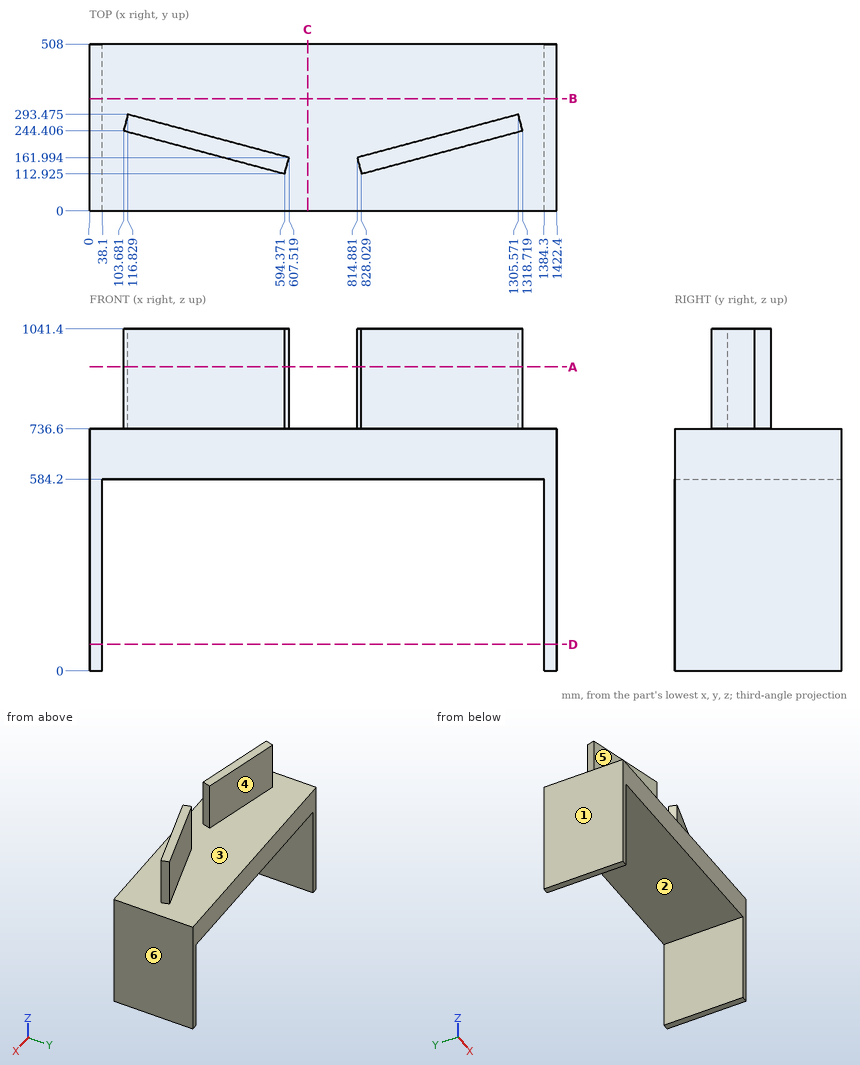
For this review, use the dimensioned drawing (mm, ordinates from the lowest corner) and the shaded views. A direction names the side the tool comes from. Round coordinates to 2 decimals unless told otherwise and drop trailing zeros. Order: outer loops, then holes, each group sorted by start corner. A loop starts at its lowest first (then second) coordinate and runs counter-clockwise, first axis right, second up. Notation, with made-up numbers: (76.25, 72) -> (94.25, 72) arc R21 cw to (94.25, 81) -> close; hole circle Ø8 at (-24, 14.25). An arc over 180 degrees is marked (long way). Use CSV: the item, a comma, the result in double quotes. Start each with the question number.
(1) Wall thickness on probe 1 along X at (y, z) = (65, 501); probe 2 along Z at (x, y) = (294, 259.5); probe 3 along Y at (x, z) = (975.5, 996): over which ranges is each line inside the solid? List them lowest first. Write a range as from..to.
(2) Insertion check: pin 1 (3 mm diameter, centred on y = 279.5, z = 882, fed in from -X); pin 2 (12 mm diameter, centred on x = 143.5, y = 300, fed in from -Z). Each pin has a flat end and moves straight along its axis. Give the tip position at first contact, or say it passes through.
(3) Consider section D-D on z = 81. Write out the cut boundary in (x, y).
(4) Consider section A-A on z = 925.5. Write out the cut boundary in (x, y) (1 decimal).
(5) Mouldability with a two-part tool opening along X and no side actions: class the marked faces 4, 5 and 6 as pulls with the +X half, pulls with the -X half, needs draft (parallel to the pull), parting line crosses it, or undercut.
(6) Consider section C-C on x = 664.5. Write out the cut boundary in (y, z), and give its area (3 significant figures).
(7) Consider section B-B on y = 341.5. Write out the cut boundary in (x, z), and give its area (3 significant figures).
(8) Tool access review of the marked faces 1, 2 and 3: name each direction out of +Z, -Z, +X, -X, +Y, -Y from which nothing blocks a thin tool from reaching the whole face with its end or side.
Responses:
1,probe 1,"0..38.1, 1384.3..1422.4"
1,probe 2,"584.2..736.6"
1,probe 3,"152.44..205.03"
2,pin 1,"x = 112.68"
2,pin 2,"z = 584.2"
3,outline,"(0, 0) -> (38.1, 0) -> (38.1, 508) -> (0, 508) -> close; (1384.3, 0) -> (1422.4, 0) -> (1422.4, 508) -> (1384.3, 508) -> close"
4,outline,"(103.7, 244.4) -> (594.4, 112.9) -> (607.5, 162) -> (116.8, 293.5) -> close; (814.9, 162) -> (828, 112.9) -> (1318.7, 244.4) -> (1305.6, 293.5) -> close"
5,face 4,"undercut"
5,face 5,"pulls with the -X half"
5,face 6,"pulls with the +X half"
6,outline,"(0, 584.2) -> (508, 584.2) -> (508, 736.6) -> (0, 736.6) -> close"
6,area,"77,400 mm²"
7,outline,"(0, 0) -> (38.1, 0) -> (38.1, 584.2) -> (1384.3, 584.2) -> (1384.3, 0) -> (1422.4, 0) -> (1422.4, 736.6) -> (0, 736.6) -> close"
7,area,"261,000 mm²"
8,face 1,"+Z, -Z, -X, +Y, -Y"
8,face 2,"-Z, +Y, -Y"
8,face 3,"+Z"
